Source: CAD feature listing. Evaluate the final solid. Frame: model axes, mm. A direction names the side the tool comes from. Give positions to 0.01 mm unless a question says otherwise; leave off trailing zeros. Order: outer loops, then holes, each group sorted by start corner. A loop starts at its lowest first (then second) coordinate and runs counter-clockwise, first axis right, second up.
1) Section D-D, the plane y = -100. Return loops of the section in (x, z) (3 decimals), plus the area to 3 significant figures.
2) Material intervals for line 1 (Y direction, x = 4, z = 2.75); line 2 (Y direction, x = -1, z = -1.75); line 3 (X direction, y = -102, z = 3), sorted ascending.
3) Section B-B, the plane y = -76.2. Return loops of the section in (x, z) (3 decimals), plus the area to 3 significant figures.
4) Section A-A, the plane z = 1.5. Give the number of separate pieces and of enclosed holes in the cut face, plus the area to 3 significant figures.
5) Access query for faces 1 (the face through (51.21, -81.974, 0.044)), 2 (the face through (-32.79, -68.81, 0.04)). Directions: +Z, -Z, +X, -X, +Y, -Y. A direction counts if a zero-diameter tool reaches every point of the face in a straight line with its end or side. Return the directions, or none.
6) First-contact query: P1, Ø3, axis at y = -83.5, z = -2, coming from the -X side; P2, Ø3, axis at x = 0.5, z = 1, coming from the -Y side. Flat tips, straight axial feed; report the tip coordinate or a pass-through.
7) Draft query along X for faces 3 (the face through (-17.96, -57.28, 0.04)), 4 (the face through (43.76, -79.3, -0.04)), 5 (the face through (-16, -67, -3.175)). Return one class per face: released by +X, released by -X, zero draft, split by the parting line, or undercut.
8) Section C-C, the plane x = 44.45. Return loops of the section in (y, z) (3 decimals), plus the area to 3 significant figures.
```python
from build123d import *

# Parameters (mm, degrees)
SKETCH1_R      = 3.175
EXTRUDE1_DEPTH = 3.175


with BuildPart() as part:
    # Sketch1 → Extrude1 (new, symmetric)
    with BuildSketch(Plane.XY):
        with BuildLine():
            Line((-30.671954233, -68.444522869), (15.048045767, -68.444522869))
            ThreePointArc((15.048045767, -68.444522869), (27.561669737, -71.74092101), (36.827271125, -80.774505929))
            ThreePointArc((36.827271125, -80.774505929), (51.362538063, -81.790073124), (47.328528799, -67.788925636))
            ThreePointArc((47.328528799, -67.788925636), (41.365390525, -65.602009691), (35.503100856, -63.157591707))
            ThreePointArc((35.503100856, -63.157591707), (-18.723497615, -57.436104054), (-66.09004738, -84.448496879))
            ThreePointArc((-66.09004738, -84.448496879), (-67.32359299, -86.435368185), (-67.754245932, -88.734026577))
            Line((-67.754245932, -88.734026577), (-67.754245932, -101.636771367))
            ThreePointArc((-67.754245932, -101.636771367), (-58.864245932, -110.526771367), (-49.974245932, -101.636771367))
            ThreePointArc((-49.974245932, -101.636771367), (-45.935885769, -83.975243651), (-34.623381697, -69.82373611))
            ThreePointArc((-34.623381697, -69.82373611), (-32.764560752, -68.799233221), (-30.671954233, -68.444522869))
        make_face()
        with Locations((44.45, -76.2)):
            Circle(SKETCH1_R, mode=Mode.SUBTRACT)
        with Locations((-58.864245932, -101.636771367)):
            Circle(SKETCH1_R, mode=Mode.SUBTRACT)
    extrude(amount=EXTRUDE1_DEPTH, both=True)


solid = part.part
```
From the geometry:
1. outline: (-67.754, -3.175) - (-61.585, -3.175) - (-61.585, 3.175) - (-67.754, 3.175) - close; (-56.144, -3.175) - (-49.941, -3.175) - (-49.941, 3.175) - (-56.144, 3.175) - close
1. area: 78.6 mm2
2. line 1: y = -68.44 to -55.66
2. line 2: y = -68.44 to -55.55
2. line 3: x = -67.75 to -62.02, -55.71 to -49.98
3. outline: (-57.46, -3.175) - (-41.029, -3.175) - (-41.029, 3.175) - (-57.46, 3.175) - close; (33.319, -3.175) - (41.275, -3.175) - (41.275, 3.175) - (33.319, 3.175) - close; (47.625, -3.175) - (53.34, -3.175) - (53.34, 3.175) - (47.625, 3.175) - close
3. area: 191 mm2
4. separate pieces: 1
4. enclosed holes: 2
4. area: 1,780 mm2
5. face 1: +Z, -Z
5. face 2: +Z, -Z, -Y
6. P1: stops at x = -66.54
6. P2: stops at y = -68.44
7. face 3: split by the parting line
7. face 4: undercut
7. face 5: zero draft
8. outline: (-85.09, -3.175) - (-79.375, -3.175) - (-79.375, 3.175) - (-85.09, 3.175) - close; (-73.025, -3.175) - (-66.77, -3.175) - (-66.77, 3.175) - (-73.025, 3.175) - close
8. area: 76.0 mm2
